Autodesk Inventor part; units mm, degrees
ref_plane "YZ Plane" through (0, 0, 0) normal (1, 0, 0) x (0, 1, 0)
ref_plane "XZ Plane" through (0, 0, 0) normal (0, 1, 0) x (-1, 0, 0)
ref_plane "XY Plane" through (0, 0, 0) normal (0, 0, 1) x (1, 0, 0)
sketch "Sketch1" plane through (0, 0, 0) normal (0, 0, 1) x (1, 0, 0)
  line L0 (100.0979, -38.5222) -> (0.0979, -38.5222)
  line L1 (0.0979, -426.5222) -> (100.0979, -426.5222)
  line L2 (82.7645, -93.1222) -> (58.7645, -93.1222)
  line L3 (58.7645, -93.1222) -> (58.7645, -101.9222)
  line L4 (58.7645, -101.9222) -> (82.7645, -101.9222)
  line L5 (82.7645, -101.9222) -> (82.7645, -93.1222)
  line L6 (41.4312, -93.1222) -> (17.4312, -93.1222)
  line L7 (17.4312, -93.1222) -> (17.4312, -101.9222)
  line L8 (17.4312, -101.9222) -> (41.4312, -101.9222)
  line L9 (41.4312, -101.9222) -> (41.4312, -93.1222)
  line L10 (38.0979, -363.1222) -> (62.0979, -363.1222)
  line L11 (62.0979, -363.1222) -> (62.0979, -371.9222)
  line L12 (62.0979, -371.9222) -> (38.0979, -371.9222)
  line L13 (38.0979, -371.9222) -> (38.0979, -363.1222)
  line L14 (173.8639, -93.5222) -> (-221.1361, -93.5222)
  line L15 (173.8639, -101.5222) -> (-221.1361, -101.5222)
  line L16 (173.8639, -371.5222) -> (-221.1361, -371.5222)
  line L17 (173.8639, -363.5222) -> (-221.1361, -363.5222)
  line L18 (34.8712, -93.1222) -> (34.8712, -93.5222) construction
  line L19 (34.8712, -101.5222) -> (34.8712, -101.9222) construction
  line L20 (58.7645, -93.1222) -> (41.4312, -93.1222) construction
  line L21 (10.9151, -363.1222) -> (10.9151, -363.5222) construction
  line L22 (10.9151, -371.5222) -> (10.9151, -371.9222) construction
  line L23 (38.0979, -363.1222) -> (12.0979, -363.1222) construction
  line L24 (62.0979, -363.1222) -> (88.0979, -363.1222) construction
  line L25 (0, 0) -> (0, -9.7735) construction
  circle A0 centre (65.5979, -390.5222) radius 1.625
  circle A1 centre (65.5979, -421.5222) radius 1.625
  circle A2 centre (34.5979, -421.5222) radius 1.625
  circle A3 centre (34.5979, -390.5222) radius 1.625
  line L26 (65.5979, -390.5222) -> (34.5979, -390.5222) construction
  line L27 (34.5979, -390.5222) -> (34.5979, -421.5222) construction
  line L28 (34.5979, -421.5222) -> (65.5979, -421.5222) construction
  line L29 (65.5979, -421.5222) -> (65.5979, -390.5222) construction
  circle A4 centre (50.0979, -406.0222) radius 12.5
  line L30 (50.0979, -390.5222) -> (50.0979, -406.0222) construction
  line L31 (50.0979, -406.0222) -> (65.5979, -406.0222) construction
  line L32 (72.2645, -85.1222) -> (80.2645, -85.1222)
  line L33 (80.2645, -85.1222) -> (80.2645, -89.1222)
  line L34 (80.2645, -89.1222) -> (72.2645, -89.1222)
  line L35 (72.2645, -89.1222) -> (72.2645, -85.1222)
  line L36 (80.2645, -89.1222) -> (82.7645, -89.1222) construction
  line L37 (82.7645, -89.1222) -> (82.7645, -93.1222) construction
  line L38 (69.2645, -85.1222) -> (61.2645, -85.1222)
  line L39 (61.2645, -85.1222) -> (61.2645, -89.1222)
  line L40 (61.2645, -89.1222) -> (69.2645, -89.1222)
  line L41 (69.2645, -89.1222) -> (69.2645, -85.1222)
  line L42 (58.7645, -93.1222) -> (58.7645, -89.1222) construction
  line L43 (58.7645, -89.1222) -> (61.2645, -89.1222) construction
  line L44 (72.2645, -105.9222) -> (80.2645, -105.9222)
  line L45 (80.2645, -105.9222) -> (80.2645, -109.9222)
  line L46 (80.2645, -109.9222) -> (72.2645, -109.9222)
  line L47 (72.2645, -109.9222) -> (72.2645, -105.9222)
  line L48 (80.2645, -105.9222) -> (80.2645, -101.9222) construction
  line L49 (69.2645, -105.9222) -> (61.2645, -105.9222)
  line L50 (61.2645, -105.9222) -> (61.2645, -109.9222)
  line L51 (61.2645, -109.9222) -> (69.2645, -109.9222)
  line L52 (69.2645, -109.9222) -> (69.2645, -105.9222)
  line L53 (38.9312, -85.1222) -> (30.9312, -85.1222)
  line L54 (30.9312, -85.1222) -> (30.9312, -89.1222)
  line L55 (30.9312, -89.1222) -> (38.9312, -89.1222)
  line L56 (38.9312, -89.1222) -> (38.9312, -85.1222)
  line L57 (27.9312, -85.1222) -> (19.9312, -85.1222)
  line L58 (19.9312, -85.1222) -> (19.9312, -89.1222)
  line L59 (19.9312, -89.1222) -> (27.9312, -89.1222)
  line L60 (27.9312, -89.1222) -> (27.9312, -85.1222)
  line L61 (30.9312, -105.9222) -> (38.9312, -105.9222)
  line L62 (38.9312, -105.9222) -> (38.9312, -109.9222)
  line L63 (38.9312, -109.9222) -> (30.9312, -109.9222)
  line L64 (30.9312, -109.9222) -> (30.9312, -105.9222)
  line L65 (27.9312, -105.9222) -> (19.9312, -105.9222)
  line L66 (19.9312, -105.9222) -> (19.9312, -109.9222)
  line L67 (19.9312, -109.9222) -> (27.9312, -109.9222)
  line L68 (27.9312, -109.9222) -> (27.9312, -105.9222)
  line L69 (41.4312, -93.1222) -> (41.4312, -89.1222) construction
  line L70 (41.4312, -89.1222) -> (38.9312, -89.1222) construction
  line L71 (17.4312, -93.1222) -> (17.4312, -89.1222) construction
  line L72 (17.4312, -89.1222) -> (19.9312, -89.1222) construction
  line L73 (51.5979, -355.1222) -> (59.5979, -355.1222)
  line L74 (59.5979, -355.1222) -> (59.5979, -359.1222)
  line L75 (59.5979, -359.1222) -> (51.5979, -359.1222)
  line L76 (51.5979, -359.1222) -> (51.5979, -355.1222)
  line L77 (48.5979, -355.1222) -> (40.5979, -355.1222)
  line L78 (40.5979, -355.1222) -> (40.5979, -359.1222)
  line L79 (40.5979, -359.1222) -> (48.5979, -359.1222)
  line L80 (48.5979, -359.1222) -> (48.5979, -355.1222)
  line L81 (51.5979, -375.9222) -> (59.5979, -375.9222)
  line L82 (59.5979, -375.9222) -> (59.5979, -379.9222)
  line L83 (59.5979, -379.9222) -> (51.5979, -379.9222)
  line L84 (51.5979, -379.9222) -> (51.5979, -375.9222)
  line L85 (48.5979, -375.9222) -> (40.5979, -375.9222)
  line L86 (40.5979, -375.9222) -> (40.5979, -379.9222)
  line L87 (40.5979, -379.9222) -> (48.5979, -379.9222)
  line L88 (48.5979, -379.9222) -> (48.5979, -375.9222)
  line L89 (59.5979, -359.1222) -> (62.0979, -359.1222) construction
  line L90 (62.0979, -359.1222) -> (62.0979, -363.1222) construction
  line L91 (38.0979, -363.1222) -> (38.0979, -359.1222) construction
  line L92 (38.0979, -359.1222) -> (40.5979, -359.1222) construction
  line L93 (59.5979, -375.9222) -> (59.5979, -371.9222) construction
  circle A5 centre (73.5979, -50.5222) radius 2.125
  circle A6 centre (26.5979, -50.5222) radius 2.125
  line L94 (73.5979, -50.5222) -> (100.0979, -50.5222) construction
  line L95 (26.5979, -50.5222) -> (0.0979, -50.5222) construction
  line L96 (96.5979, -57.5222) -> (88.5979, -57.5222)
  line L97 (11.5979, -57.5222) -> (3.5979, -57.5222)
  line L98 (8.0979, -43.5222) -> (8.0979, -57.5222)
  line L99 (7.0979, -57.5222) -> (7.0979, -43.5222)
  line L100 (93.0979, -43.5222) -> (93.0979, -57.5222)
  line L101 (92.0979, -57.5222) -> (92.0979, -43.5222)
  line L102 (7.5979, -57.5222) -> (7.5979, -426.5222) construction
  line L103 (92.5979, -57.5222) -> (92.5979, -426.5222) construction
  circle A7 centre (92.5979, -419.5222) radius 2.125
  circle A8 centre (92.5979, -392.5222) radius 2.125
  circle A9 centre (7.5979, -419.5222) radius 2.125
  circle A10 centre (7.5979, -392.5222) radius 2.125
  line L104 (92.5979, -419.5222) -> (7.5979, -419.5222) construction
  line L105 (92.5979, -392.5222) -> (7.5979, -392.5222) construction
  line L106 (100.0979, -38.5222) -> (100.0979, -81.5222)
  line L107 (100.0979, -81.5222) -> (88.0979, -81.5222)
  line L108 (88.0979, -81.5222) -> (88.0979, -113.5222)
  line L109 (88.0979, -113.5222) -> (100.0979, -113.5222)
  line L110 (100.0979, -351.5222) -> (88.0979, -351.5222)
  line L111 (88.0979, -351.5222) -> (88.0979, -383.5222)
  line L112 (88.0979, -383.5222) -> (100.0979, -383.5222)
  line L113 (100.0979, -383.5222) -> (100.0979, -426.5222)
  line L114 (100.0979, -81.5222) -> (100.0979, -93.5222) construction
  line L115 (100.0979, -101.5222) -> (100.0979, -113.5222) construction
  line L116 (0.0979, -38.5222) -> (0.0979, -81.5222)
  line L117 (0.0979, -81.5222) -> (12.0979, -81.5222)
  line L118 (12.0979, -81.5222) -> (12.0979, -113.5222)
  line L119 (12.0979, -113.5222) -> (0.0979, -113.5222)
  line L120 (0.0979, -351.5222) -> (12.0979, -351.5222)
  line L121 (12.0979, -351.5222) -> (12.0979, -383.5222)
  line L122 (12.0979, -383.5222) -> (0.0979, -383.5222)
  line L123 (0.0979, -383.5222) -> (0.0979, -426.5222)
  line L124 (98.1469, -351.5222) -> (98.1469, -363.5222) construction
  line L125 (98.1469, -383.5222) -> (98.1469, -371.5222) construction
  line L126 (17.4312, -93.1222) -> (12.0979, -93.1222) construction
  line L127 (82.7645, -93.1222) -> (88.0979, -93.1222) construction
  line L128 (82.7645, -97.5222) -> (100.0979, -97.5222) construction
  line L129 (58.7645, -97.5222) -> (41.4312, -97.5222) construction
  line L130 (17.4312, -97.5222) -> (0.0979, -97.5222) construction
  line L131 (38.0979, -367.5222) -> (0.0979, -367.5222) construction
  line L132 (62.0979, -367.5222) -> (100.0979, -367.5222) construction
  line L133 (100.0979, -113.5222) -> (100.0979, -207.5222)
  line L134 (100.0979, -207.5222) -> (88.0979, -207.5222)
  line L135 (88.0979, -207.5222) -> (88.0979, -257.5222)
  line L136 (88.0979, -257.5222) -> (100.0979, -257.5222)
  line L137 (100.0979, -257.5222) -> (100.0979, -351.5222)
  line L138 (0.0979, -113.5222) -> (0.0979, -207.5222)
  line L139 (0.0979, -207.5222) -> (12.0979, -207.5222)
  line L140 (12.0979, -207.5222) -> (12.0979, -257.5222)
  line L141 (12.0979, -257.5222) -> (0.0979, -257.5222)
  line L142 (0.0979, -257.5222) -> (0.0979, -351.5222)
  line L143 (34.5979, -390.5222) -> (0.0979, -390.5222) construction
  line L144 (65.5979, -390.5222) -> (100.0979, -390.5222) construction
  circle A11 centre (40.0979, -232.5222) radius 2.125
  circle A12 centre (60.0979, -232.5222) radius 2.125
  line L145 (40.0979, -232.5222) -> (60.0979, -232.5222) construction
  line L146 (40.0979, -232.5222) -> (12.0979, -232.5222) construction
  line L147 (60.0979, -232.5222) -> (88.0979, -232.5222) construction
  dimension "d1" = 24
  dimension "d2" = 8.8
  dimension "d3" = 100
  dimension "d9" = 55
  dimension "d10" = 55
  dimension "d11" = 3.25
  dimension "d12" = 31
  dimension "d13" = 5
  dimension "d14" = 25
  dimension "d15" = 4
  dimension "d16" = 8
  dimension "d17" = 4
  dimension "d18" = 2.5
  dimension "d19" = 4.25
  dimension "d20" = 4.25
  dimension "d21" = 47
  dimension "d22" = 12
  dimension "d23" = 4.25
  dimension "d24" = 4.25
  dimension "d25" = 27
  dimension "d26" = 7
  dimension "d27" = 4.25
  dimension "d28" = 4.25
  dimension "d29" = 32
  dimension "d30" = 12
  dimension "d31" = 50
  dimension "d32" = 4.25
  dimension "d33" = 4.25
  dimension "d34" = 20
  dimension "d35" = 25
extrude "Extrusion1" add sketch "Sketch1" along normal blind 5 contours L106 L107 L108 L14 L5 L2 L3 L9 L6 L7 L118 L117 L116 L0 | L108 L15 L5 L14 | L14 L7 L15 L118 | L108 L109 L133 L134 L135 L136 L137 L110 L111 L17 L11 L10 L13 L121 L120 L142 L141 L140 L139 L138 L119 L118 L15 L7 L8 L9 L3 L4 L5 | L3 L15 L9 L14 | L111 L16 L11 L17 | L17 L13 L16 L121 | L111 L112 L113 L1 L123 L122 L121 L16 L13 L12 L11
sketch "Sketch2" plane through (17.4312, -101.9222, 0) normal (1, 0, 0) x (0, 0, -1)
  circle A0 centre (6.0737, 4.4) radius 7.5
  point P0 (0, 101.9222)
  point P1 (0, 8.8)
  point P2 (0, 0)
  dimension "d6" = 15
sketch "Sketch3" plane through (38.0979, -371.9222, 0) normal (1, 0, 0) x (0, 0, -1)
  circle A0 centre (6.0737, 4.4) radius 7.5
  point P0 (0, 371.9222)
  point P1 (0, 8.8)
  point P2 (0, 0)
  dimension "d8" = 15
properties part number "XCartFloor"
Work out the finished part from the listing and answer in its coordinate system (mm). Coordinates: 2 decimals unless noted, no trailing zeros. Write each loop counter-clockwise with the first axis right and the second up, starting at its lowest first coordinate (ties: lowest second). Pieces come first, ordered by that corner, then holes. Notation, with made-up numbers: (-20, -3) - (20, -3) arc R37 cw to (20, 35) - close; hole circle Ø10 at (26, -6). An arc over 180 degrees is marked (long way). Answer as a JSON object with one key per item and string values.
Q1. For a pull along X with two mould halves and no side action, classify faces 1 (the cylindrical face through (48.471, -418.416, 2.465)), 2 (the flat face through (49, -230, 0)) as pulls with the +X half, pulls with the -X half, needs draft (parallel to the pull), parting line crosses it, or undercut.
Results list:
{"face 1": "undercut", "face 2": "needs draft"}
Q2. Find section A-A (y = -248). Write down the section's boundary in (x, z).
Results list:
{"outline": "(12.1, 0) - (88.1, 0) - (88.1, 5) - (12.1, 5) - close"}
Q3. Find section B-B (z = 3.3). State how many separate pieces and enclosed holes the cut face has, plus the area to 3 significant figures.
Results list:
{"separate pieces": "1", "enclosed holes": "28", "area": "34,400 mm^2"}
Q4. Given pin 1 Ø2 at (y, z) = (-87, 3) entering from -X; pin 2 Ø1.2 at (y, z) = (-86.5, 3) entering from +X, each flat-ended and moving along its own axis, determine where each tip first touches the part or whether it passes through.
Results list:
{"pin 1": "stops at x = 12.1", "pin 2": "stops at x = 88.1"}
Q5. Consider L1, parallel to Y at x = 68.5, z = 4.2; L2, parallel to Y at x = 49.5, z = 2.2; L3, parallel to Y at x = 92, z = 1.2. Determine where each line is inside the solid, lowest interval first. Write a range as from..to.
Results list:
{"L1": "y = -426.52..-109.92, -105.92..-101.92, -93.12..-89.12, -85.12..-38.52", "L2": "y = -426.52..-418.51, -393.54..-371.92, -363.12..-38.52", "L3": "y = -426.52..-421.56, -417.48..-394.56, -390.48..-383.52, -351.52..-257.52, -207.52..-113.52, -81.52..-38.52"}
